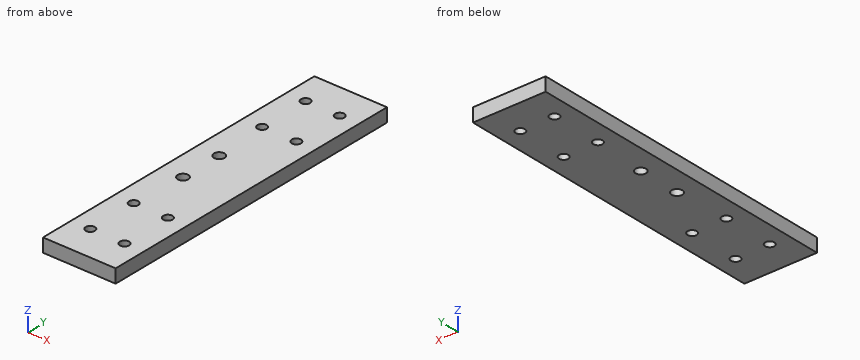
```python
from build123d import *

# Parameters (mm, degrees)
SKETCH1_W              = 34
SKETCH1_H              = 150
BOSS_EXTRUDE1_DEPTH    = 6.35
F_8_CLEARANCE_HOLE1_D  = 4.3053
F_10_CLEARANCE_HOLE1_D = 4.9784


with BuildPart() as part:
    # Sketch1 → Boss-Extrude1 (new body)
    with BuildSketch(Plane.XY):
        Rectangle(SKETCH1_W, SKETCH1_H)
    extrude(amount=BOSS_EXTRUDE1_DEPTH)

    # #8 Clearance Hole1 (through all)
    with Locations(Plane.XY.offset(6.35)):
        with Locations((-8, 59.5), (8, 59.5), (8, 35.5), (-8, 35.5), (-8, -35.5), (-8, -59.5), (8, -59.5), (8, -35.5)):
            Hole(F_8_CLEARANCE_HOLE1_D / 2)

    # #10 Clearance Hole1 (through all)
    with Locations(Plane.XY.offset(6.35)):
        with Locations((-6.5, 10), (-6.5, -10)):
            Hole(F_10_CLEARANCE_HOLE1_D / 2)


solid = part.part
```
Check sheet for the modelled part. Datum: model origin and axes. Units: mm. Give positions to 0.01 mm unless a question says otherwise; leave off trailing zeros. Write each loop counter-clockwise with the first axis right and the second up, starting at its lowest first coordinate (ties: lowest second). Pieces come first, ordered by that corner, then holes. Notation, with made-up numbers: (-38.5, 6) - (-1.5, 6) arc R25 ccw to (-1.5, 44) - close; hole circle Ø5 at (12, 77). An arc over 180 degrees is marked (long way). Answer as a JSON object with one key per item and string values. Group by question number.
1) Sectioned sample at B-B (x = 8). Record the cut outline in (y, z).
2) Thickness scan on probe 1 along Y at (x, z) = (8, 2.5); probe 2 along Y at (x, z) = (-4.5, 0.5); probe 3 along X at (y, z) = (-36.5, 1). Record the ranges inside material, lowest first. Write a range as from..to.
3) Sectioned sample at C-C (z = 2). Give the number of separate pieces and of enclosed holes in the cut face, then the cut area to 3 significant figures.
4) Sectioned sample at D-D (y = 35.5). Record the cut outline in (x, z).
5) Depth check by flat-ended pin: P1, Ø4.5, axis at x = -6.5, y = 10, coming from the +Z side. Enter the tip coordinate at first touch or a pass-through.
6) Sectioned sample at A-A (y = 10). Record the cut outline in (x, z), then the cut area to 3 significant figures.
Geometry results:
{
 "1": {"outline": "(-75, 0) - (-61.65, 0) - (-61.65, 6.35) - (-75, 6.35) - close; (-57.35, 0) - (-37.65, 0) - (-37.65, 6.35) - (-57.35, 6.35) - close; (-33.35, 0) - (33.35, 0) - (33.35, 6.35) - (-33.35, 6.35) - close; (37.65, 0) - (57.35, 0) - (57.35, 6.35) - (37.65, 6.35) - close; (61.65, 0) - (75, 0) - (75, 6.35) - (61.65, 6.35) - close"},
 "2": {"probe 1": "y = -75..-61.65, -57.35..-37.65, -33.35..33.35, 37.65..57.35, 61.65..75", "probe 2": "y = -75..-11.48, -8.52..8.52, 11.48..75", "probe 3": "x = -17..-9.91, -6.09..6.09, 9.91..17"},
 "3": {"separate pieces": "1", "enclosed holes": "10", "area": "4,940 mm^2"},
 "4": {"outline": "(-17, 0) - (-10.15, 0) - (-10.15, 6.35) - (-17, 6.35) - close; (-5.85, 0) - (5.85, 0) - (5.85, 6.35) - (-5.85, 6.35) - close; (10.15, 0) - (17, 0) - (17, 6.35) - (10.15, 6.35) - close"},
 "5": {"P1": "passes through"},
 "6": {"outline": "(-17, 0) - (-8.99, 0) - (-8.99, 6.35) - (-17, 6.35) - close; (-4.01, 0) - (17, 0) - (17, 6.35) - (-4.01, 6.35) - close", "area": "184 mm^2"}
}
